```python
from build123d import *

# Parameters (mm, degrees)
SKETCH1_R           = 4.5
BOSS_EXTRUDE1_DEPTH = 3.5
SKETCH2_W           = 15
SKETCH2_H           = 3.5
CUT_EXTRUDE1_DEPTH  = 45.343122353


with BuildPart() as part:
    # Sketch1 → Boss-Extrude1 (new body)
    with BuildSketch(Plane.XY):
        Polygon((27.25, -26), (27.25, -22.5), (32.25, -22.5), (32.25, -11), (35.75, -11), (35.75, -7.5), (32.25, -7.5), (32.25, 7.5), (35.75, 7.5), (35.75, 11), (32.25, 11), (32.25, 22.5), (27.25, 22.5), (27.25, 26), (12.25, 26), (12.25, 22.5), (-12.25, 22.5), (-12.25, 26), (-27.25, 26), (-27.25, 22.5), (-32.25, 22.5), (-32.25, -22.5), (-27.25, -22.5), (-27.25, -26), (-12.25, -26), (-12.25, -22.5), (12.25, -22.5), (12.25, -26), align=None)
        Circle(SKETCH1_R, mode=Mode.SUBTRACT)
        with BuildLine():
            Line((-11.277098909, -7.667491727), (-5.734536325, -4.467491727))
            ThreePointArc((-5.734536325, -4.467491727), (-5.36789118, -3.099153418), (-6.736229489, -2.732508273))
            Line((-6.736229489, -2.732508273), (-12.278792074, -5.932508273))
            ThreePointArc((-12.278792074, -5.932508273), (-12.645437219, -7.300846582), (-11.277098909, -7.667491727))
        make_face(mode=Mode.SUBTRACT)
        with BuildLine():
            Line((1, 19), (1, 7))
            ThreePointArc((1, 7), (0, 6), (-1, 7))
            Line((-1, 7), (-1, 19))
            ThreePointArc((-1, 19), (0, 20), (1, 19))
        make_face(mode=Mode.SUBTRACT)
        with BuildLine():
            Line((-12.278792074, 5.932508273), (-6.736229489, 2.732508273))
            ThreePointArc((-6.736229489, 2.732508273), (-5.36789118, 3.099153418), (-5.734536325, 4.467491727))
            Line((-5.734536325, 4.467491727), (-11.277098909, 7.667491727))
            ThreePointArc((-11.277098909, 7.667491727), (-12.645437219, 7.300846582), (-12.278792074, 5.932508273))
        make_face(mode=Mode.SUBTRACT)
        with BuildLine():
            Line((11.277098909, 7.667491727), (5.734536325, 4.467491727))
            ThreePointArc((5.734536325, 4.467491727), (5.36789118, 3.099153418), (6.736229489, 2.732508273))
            Line((6.736229489, 2.732508273), (12.278792074, 5.932508273))
            ThreePointArc((12.278792074, 5.932508273), (12.645437219, 7.300846582), (11.277098909, 7.667491727))
        make_face(mode=Mode.SUBTRACT)
        with BuildLine():
            Line((12.278792074, -5.932508273), (6.736229489, -2.732508273))
            ThreePointArc((6.736229489, -2.732508273), (5.36789118, -3.099153418), (5.734536325, -4.467491727))
            Line((5.734536325, -4.467491727), (11.277098909, -7.667491727))
            ThreePointArc((11.277098909, -7.667491727), (12.645437219, -7.300846582), (12.278792074, -5.932508273))
        make_face(mode=Mode.SUBTRACT)
        with BuildLine():
            Line((1, -19), (1, -7))
            ThreePointArc((1, -7), (0, -6), (-1, -7))
            Line((-1, -7), (-1, -19))
            ThreePointArc((-1, -19), (0, -20), (1, -19))
        make_face(mode=Mode.SUBTRACT)
    extrude(amount=BOSS_EXTRUDE1_DEPTH)

    # Sketch2 → Cut-Extrude1 (cut, through all)
    with BuildSketch(Plane(origin=(0, 0, 0), x_dir=(-1, 0, 0), z_dir=(0, 0, -1))):
        with Locations((19.65, -0.25)):
            Rectangle(SKETCH2_W, SKETCH2_H)
        with Locations((-19.75, -0.25)):
            Rectangle(SKETCH2_W, SKETCH2_H)
    extrude(amount=-CUT_EXTRUDE1_DEPTH, mode=Mode.SUBTRACT)


solid = part.part
```
Can you work these out from the model? Positions are in its coordinate system, mm. A direction names the side the tool comes from. Coordinates: 2 decimals unless noted, no trailing zeros. Loops run counter-clockwise (first coordinate to the right, second up) from the corner with the lowest first, then second, coordinate; pieces in that order, holes last. Notation, with made-up numbers: (-37, 72) - (-10, 72) arc R36 ccw to (-10, 108) - close; hole circle Ø2 at (-14, 33). An arc over 180 degrees is marked (long way). Use a Markdown table: item, result.
Item 1: If I drill on probe 1 along Y at (x, z) = (0, 2.4); probe 2 along X at (y, z) = (8.5, 1.85); probe 3 along X at (y, z) = (13.5, 0.3), over which ranges is the centre line in solid material (lowest first)? Write a range as from..to.
Numbers:
| item | result |
|---|---|
| probe 1 | y = -22.5..-20, -6..-4.5, 4.5..6, 20..22.5 |
| probe 2 | x = -32.25..-1, 1..35.75 |
| probe 3 | x = -32.25..-1, 1..32.25 |
Item 2: For faces 1 (the face through (-12.25, -24, 2)), 2 (the face through (0, -6, 2)), 3 (the face through (-27.25, 24, 2)), 4 (the face through (32.25, -17, 2)), which set-ups out of +Z, -Z, +X, -X, +Y, -Y let a thin tool reach every point of the face, with its end or its side?
Numbers:
| item | result |
|---|---|
| face 1 | +Z, -Z, -Y |
| face 2 | +Z, -Z |
| face 3 | +Z, -Z, -X, +Y |
| face 4 | +Z, -Z, +X, -Y |
Item 3: I want a section at D-D on x = 0. Please give me the cut outline in (y, z), and give its area (3 significant figures).
Numbers:
| item | result |
|---|---|
| outline | (-22.5, 0) - (-20, 0) - (-20, 3.5) - (-22.5, 3.5) - close; (-6, 0) - (-4.5, 0) - (-4.5, 3.5) - (-6, 3.5) - close; (4.5, 0) - (6, 0) - (6, 3.5) - (4.5, 3.5) - close; (20, 0) - (22.5, 0) - (22.5, 3.5) - (20, 3.5) - close |
| area | 28.0 mm2 |
Item 4: Will these pins go through, and if not, where does the flat tip stop? pin 1 (1 mm diameter, centred on y = -15, z = 1, fed in from +X); pin 2 (1.8 mm diameter, centred on x = 2.5, z = 1.5, fed in from -Y); pin 3 (1 mm diameter, centred on y = 23.5, z = 2, fed in from +X).
Numbers:
| item | result |
|---|---|
| pin 1 | stops at x = 32.25 |
| pin 2 | stops at y = -22.5 |
| pin 3 | stops at x = 27.25 |
Item 5: We'd pull the mould along Y, two halves only. Please class faces 5 (the face through (-30, -22.5, 2)), 6 (the face through (-8.467, 6.045, 1.726)), 7 (the face through (27.25, 24, 2)): released by +Y, released by -Y, zero draft, split by the parting line, or undercut.
Numbers:
| item | result |
|---|---|
| face 5 | released by -Y |
| face 6 | undercut |
| face 7 | zero draft |
Item 6: I want a section at A-A on y = 0. Please give me the cut outline in (x, z), and give its area (4 significant figures).
Numbers:
| item | result |
|---|---|
| outline | (-32.25, 0) - (-27.15, 0) - (-27.15, 3.5) - (-32.25, 3.5) - close; (-12.15, 0) - (-4.5, 0) - (-4.5, 3.5) - (-12.15, 3.5) - close; (4.5, 0) - (12.25, 0) - (12.25, 3.5) - (4.5, 3.5) - close; (27.25, 0) - (32.25, 0) - (32.25, 3.5) - (27.25, 3.5) - close |
| area | 89.25 mm2 |
Item 7: I want a section at B-B on x = 19.5. Please give me the cut outline in (y, z), and give its area (3 significant figures).
Numbers:
| item | result |
|---|---|
| outline | (-26, 0) - (-2, 0) - (-2, 3.5) - (-26, 3.5) - close; (1.5, 0) - (26, 0) - (26, 3.5) - (1.5, 3.5) - close |
| area | 170 mm2 |
Item 8: I want a section at C-C on y = -13. Please give me the cut outline in (x, z).
Numbers:
| item | result |
|---|---|
| outline | (-32.25, 0) - (-1, 0) - (-1, 3.5) - (-32.25, 3.5) - close; (1, 0) - (32.25, 0) - (32.25, 3.5) - (1, 3.5) - close |
